The listing builds one solid part. Answer for the finished solid, in the listing's coordinates (mm). A direction names the side the tool comes from. Coordinates: 2 decimals unless noted, no trailing zeros. Order: outer loops, then holes, each group sorted by start corner. A loop starts at its lowest first (then second) coordinate and runs counter-clockwise, first axis right, second up. Notation, with made-up numbers: (22, 50.5) -> (75, 50.5) arc R11 cw to (75, 69.5) -> close; hole circle Ø1 at (18.5, 1). An arc over 180 degrees is marked (long way). Answer in a Markdown table with one row per item.
```python
from build123d import *

# Parameters (mm, degrees)
BOSS_EXTRUDE2_DEPTH         = 4
M5_TAPPED_HOLE3_D           = 4.2
M5_TAPPED_HOLE3_CSINK_D     = 5.05
M5_TAPPED_HOLE3_CSINK_ANGLE = 90


with BuildPart() as part:
    # Sketch8 → Boss-Extrude2 (new body)
    with BuildSketch(Plane(origin=(0, 0, 0), x_dir=(1, 0, 0), z_dir=(0, 1, 0))):
        Polygon((2.400826816, -3.945803332), (4.617579332, 0.106275347), (2.216752516, 4.052078679), (-2.400826816, 3.945803332), (-4.617579332, -0.106275347), (-2.216752516, -4.052078679), align=None)
    extrude(amount=BOSS_EXTRUDE2_DEPTH)

    # M5 Tapped Hole3 (through all)
    with Locations(Plane(origin=(-0.132343684, 4, 0.02883036), x_dir=(0, 0, 1), z_dir=(0, 1, 0))):
        with Locations((0, 0), (-0.009914208, 0.154917862)):
            CounterSinkHole(M5_TAPPED_HOLE3_D / 2, M5_TAPPED_HOLE3_CSINK_D / 2, counter_sink_angle=M5_TAPPED_HOLE3_CSINK_ANGLE)


solid = part.part
```
(1) A cutting plane is placed at B-B, the plane x = -3.5. Determine the outline of the cut face in (y, z).
Check values:
| item | result |
|---|---|
| outline | (0, -1.94) -> (4, -1.94) -> (4, 1.94) -> (0, 1.94) -> close |
(2) A cutting plane is placed at A-A, the plane y = 1.2. Determine the outline of the cut face in (x, z).
Check values:
| item | result |
|---|---|
| outline | (-4.62, 0.11) -> (-2.4, -3.95) -> (2.22, -4.05) -> (4.62, -0.11) -> (2.4, 3.95) -> (-2.22, 4.05) -> close; hole (-0.19, -2.07) arc R2.1 ccw (long way) to (0.08, 2.12) arc R2.1 ccw (long way) to start |
(3) Find the intervals of material crossed by line 1 along Z through (x, y) = (1.75, 1.25); line 2 along Z through (x, y) = (0.25, 1.3); line 3 along X through (y, z) = (3.25, -1.25), in increasing order. Write a range as from..to.
Check values:
| item | result |
|---|---|
| line 1 | -4.04..-1.18, 1.21..3.96 |
| line 2 | -4.01..-2.07, 2.11..4 |
| line 3 | -3.88..-1.8, 1.7..3.92 |
(4) Which of the six approach directions +Z, -Z, +X, -X, +Y, -Y give full straight-line access (tool end or side, diameter ignored) to faces 1 (the flat face through (-3.494, 1.972, -1.948)), 2 (the cylindrical face through (-2.225, 1.762, 0.21))?
Check values:
| item | result |
|---|---|
| face 1 | -Z, -X, +Y, -Y |
| face 2 | +Y, -Y |
(5) A cutting plane is placed at C-C, the plane z = -3.5. Determine the outline of the cut face in (x, y).
Check values:
| item | result |
|---|---|
| outline | (-2.64, 0) -> (2.55, 0) -> (2.55, 4) -> (-2.64, 4) -> close |
(6) For a pull along Z with two mould halves and no side action, classify faces 3 (the flat face through (3.434, 1.972, -2.052)), 4 (the conical face through (2.23, 3.69, -0.17)), 5 (the flat face through (2, 0, 2)), 6 (the conical face through (-2.34, 3.69, 0.22)) as released by +Z, released by -Z, zero draft, split by the parting line, or undercut.
Check values:
| item | result |
|---|---|
| face 3 | released by -Z |
| face 4 | undercut |
| face 5 | zero draft |
| face 6 | undercut |
(7) Flat-ended cylindrical pins translate along their axes: pin 1 (1 mm diameter, centred on y = 3.5, z = 2.5, fed in from -X); pin 2 (2 mm diameter, centred on y = 3, z = -1, fed in from -X); pin 3 (1 mm diameter, centred on x = 1.5, y = 2.5, fed in from -Z). Find the tip coordinate at first contact, or state that the pin passes through.
Check values:
| item | result |
|---|---|
| pin 1 | x = -3.47 |
| pin 2 | x = -4.56 |
| pin 3 | z = -4.05 |
